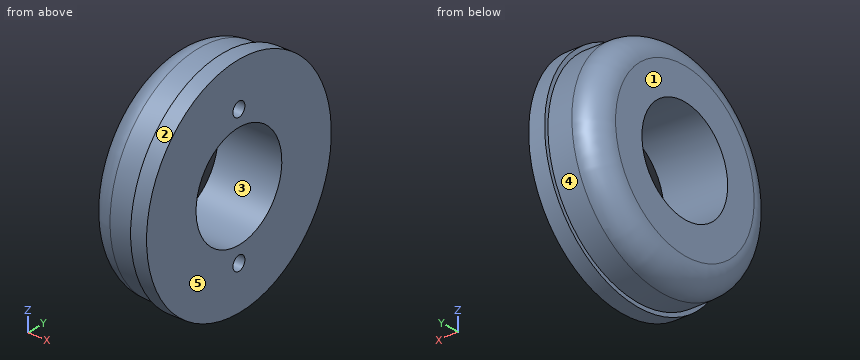
```python
from build123d import *

# Parameters (mm, degrees)
CYLINDER055_R           = 6.5
CYLINDER055_DEPTH       = 10
CYLINDER055_PITCH_ANGLE = 90
CYLINDER108_R           = 0.9
CYLINDER108_DEPTH       = 7
CYLINDER108_PITCH_ANGLE = 90
CYLINDER107_R           = 0.9
CYLINDER107_DEPTH       = 7
CYLINDER107_PITCH_ANGLE = 90
CYLINDER058_R           = 13.5
CYLINDER058_DEPTH       = 6
CYLINDER058_PITCH_ANGLE = 90
CYLINDER011_R           = 14
CYLINDER011_DEPTH       = 2
CYLINDER011_PITCH_ANGLE = 90
FILLET038_R             = 3


with BuildPart() as cylinder055:
    # Cylinder055 → Cylinder055 (new body)
    with BuildSketch(Plane.XY):
        Circle(CYLINDER055_R)
    extrude(amount=CYLINDER055_DEPTH)


with BuildPart() as cylinder055_1:
    # Cylinder055 pitch: moved
    add(cylinder055.part.rotate(Axis((0, 0, 0), (0, 1, 0)), CYLINDER055_PITCH_ANGLE))


with BuildPart() as cylinder055_2:
    # Cylinder055 placement: moved
    add(cylinder055_1.part.moved(Location((-10, 15, 27))))


with BuildPart() as cylinder108:
    # Cylinder108 → Cylinder108 (new body)
    with BuildSketch(Plane.XY):
        Circle(CYLINDER108_R)
    extrude(amount=CYLINDER108_DEPTH)


with BuildPart() as cylinder108_1:
    # Cylinder108 pitch: moved
    add(cylinder108.part.rotate(Axis((0, 0, 0), (0, 1, 0)), CYLINDER108_PITCH_ANGLE))


with BuildPart() as cylinder108_2:
    # Cylinder108 placement: moved
    add(cylinder108_1.part.moved(Location((-7, 15, 35.5))))


with BuildPart() as fusion056:
    # Cylinder107 → Cylinder107 (new body)
    with BuildSketch(Plane.XY):
        Circle(CYLINDER107_R)
    extrude(amount=CYLINDER107_DEPTH)


with BuildPart() as fusion056_1:
    # Cylinder107 pitch: moved
    add(fusion056.part.rotate(Axis((0, 0, 0), (0, 1, 0)), CYLINDER107_PITCH_ANGLE))


with BuildPart() as fusion056_2:
    # Cylinder107 placement: moved
    add(fusion056_1.part.moved(Location((-7, 15, 18.5))))

    # Fusion056: union Cylinder055, Cylinder108
    add(cylinder055_2.part)
    add(cylinder108_2.part)


with BuildPart() as cylinder058:
    # Cylinder058 → Cylinder058 (new body)
    with BuildSketch(Plane.XY):
        Circle(CYLINDER058_R)
    extrude(amount=CYLINDER058_DEPTH)


with BuildPart() as cylinder058_1:
    # Cylinder058 pitch: moved
    add(cylinder058.part.rotate(Axis((0, 0, 0), (0, 1, 0)), CYLINDER058_PITCH_ANGLE))


with BuildPart() as cylinder058_2:
    # Cylinder058 placement: moved
    add(cylinder058_1.part.moved(Location((-8, 15, 27))))


with BuildPart() as clutch_part:
    # Cylinder011 → Cylinder011 (new body)
    with BuildSketch(Plane.XY):
        Circle(CYLINDER011_R)
    extrude(amount=CYLINDER011_DEPTH)


with BuildPart() as clutch_part_1:
    # Cylinder011 pitch: moved
    add(clutch_part.part.rotate(Axis((0, 0, 0), (0, 1, 0)), CYLINDER011_PITCH_ANGLE))


with BuildPart() as clutch_part_2:
    # Cylinder011 placement: moved
    add(clutch_part_1.part.moved(Location((-2, 15, 27))))

    # Fusion029: union Cylinder058
    add(cylinder058_2.part)

    # Cut047: cut Fusion056
    add(fusion056_2.part, mode=Mode.SUBTRACT)

    # Fillet038
    fillet038_edges = [clutch_part_2.edges().sort_by_distance(p)[0] for p in [
        (-8, 15, 40.5),
    ]]
    fillet(fillet038_edges, radius=FILLET038_R)


solid = clutch_part_2.part
```
Geometry check sheet. Reference: the model listing, model coordinates, mm. Face numbers are marked on the shaded views. A direction names the side the tool comes from. Give positions to 0.01 mm unless a question says otherwise; leave off trailing zeros. Order: outer loops, then holes, each group sorted by start corner. A loop starts at its lowest first (then second) coordinate and runs counter-clockwise, first axis right, second up. Notation, with made-up numbers: (-30.75, -30.5) -> (9.25, -30.5) arc R9 cw to (9.25, -21.5) -> close; hole circle Ø2 at (10, -25.75). An arc over 180 degrees is marked (long way). Write each question's results on one line, items separated by ' | '. Start each with the question number.
(1) Mould release check, pull along Y, two halves, no side actions. Record for the marked faces 1, 2 and 3: pulls with the +Y half, pulls with the -Y half, needs draft (parallel to the pull), parting line crosses it, or undercut.
(2) Sectioned sample at D-D (x = -6.5). Enter the section's corners in (y, z), plus the area to 3 significant figures.
(3) Scan lines: line 1 (Y direction, x = -5.75, z = 27); line 2 (Y direction, x = -4, z = 28); line 3 (Z direction, x = -3, y = 13.25). Record each from-to range of solid material in increasing order.
(4) Sectioned sample at C-C (x = -3). Enter the section's corners in (y, z).
(5) Sectioned sample at B-B (y = 15). Enter the section's corners in (x, z).
(6) Access from +Z, -Z, +X, -X, +Y, -Y to the whole of each face (thin tool, end or side, straight path). Record for the marked faces 4 and 5.
(7) Sectioned sample at A-A (z = 27). Enter the section's corners in (x, y), plus the area to 3 significant figures.
(8) Gauge pin test, flat ends, axial feed: P1, Ø3, axis at x = -6, y = 13.5, coming from the -Z side; P2, Ø3, axis at x = -5.5, z = 31.5, coming from the +Y side; P3, Ø0.9, axis at y = 14.5, z = 35.5, coming from the +X side; P4, Ø4, axis at x = -7, y = 11, coming from the -Z side. Record the tip position at first contact, or that the pin passes through.
Answer below:
1) face 1: needs draft | face 2: parting line crosses it | face 3: undercut
2) outline: circle Ø26.2 at (15, 27); hole circle Ø13 at (15, 27); hole circle Ø1.8 at (15, 18.5); hole circle Ø1.8 at (15, 35.5) | area: 401 mm2
3) line 1: 1.6 to 8.5, 21.5 to 28.4 | line 2: 1.54 to 8.58, 21.42 to 28.46 | line 3: 13.61 to 20.74, 33.26 to 40.39
4) outline: circle Ø27 at (15, 27); hole circle Ø13 at (15, 27); hole circle Ø1.8 at (15, 18.5); hole circle Ø1.8 at (15, 35.5)
5) outline: (-8, 16.5) arc R3 ccw to (-5, 13.5) -> (-2, 13.5) -> (-2, 13) -> (0, 13) -> (0, 17.6) -> (-7, 17.6) -> (-7, 19.4) -> (0, 19.4) -> (0, 20.5) -> (-8, 20.5) -> close; (-8, 33.5) -> (0, 33.5) -> (0, 34.6) -> (-7, 34.6) -> (-7, 36.4) -> (0, 36.4) -> (0, 41) -> (-2, 41) -> (-2, 40.5) -> (-5, 40.5) arc R3 ccw to (-8, 37.5) -> close
6) face 4: -X | face 5: +Z, -Z, +X, +Y, -Y
7) outline: (-8, 4.5) arc R3 ccw to (-5, 1.5) -> (-2, 1.5) -> (-2, 1) -> (0, 1) -> (0, 8.5) -> (-8, 8.5) -> close; (-8, 21.5) -> (0, 21.5) -> (0, 29) -> (-2, 29) -> (-2, 28.5) -> (-5, 28.5) arc R3 ccw to (-8, 25.5) -> close | area: 110 mm2
8) P1: z = 13.5 | P2: y = 28.15 | P3: x = 0 | P4: z = 13.81
